Geometry: final body of the model. Coordinates: model frame, mm. Face numbers are marked on the shaded views. A direction names the side the tool comes from. Round coordinates to 2 decimals unless told otherwise and drop trailing zeros. Write each loop counter-clockwise with the first axis right and the second up, starting at its lowest first coordinate (ties: lowest second). Pieces come first, ordered by that corner, then holes. Notation, with made-up numbers: M 63.25,22.5 L 107.25,22.5 A13 cw 107.25,32.5 Z; hole C 55.5,44 d10. An arc over 180 degrees is marked long. Put each result on its own line as item: value. Start each with the question number.
```python
from build123d import *

# Parameters (mm, degrees)
F0_W     = 6
F0_H     = 18
F1_DEPTH = 12
F2_W     = 6
F2_H     = 9
F2_W_2   = 2
F2_H_2   = 4
F3_DEPTH = 10
F4_R     = 1.5
F5_DEPTH = 5


with BuildPart() as f1:
    # F0 (on Top) → F1 (new body)
    with BuildSketch(Plane.XY):
        Rectangle(F0_W, F0_H)
    extrude(amount=F1_DEPTH)

    # F2 (on face) → F3 (cut)
    with BuildSketch(Plane(origin=(0, 0, 0), x_dir=(1, 0, 0), z_dir=(0, 0, -1))):
        with Locations((0, 4.5)):
            Rectangle(F2_W, F2_H)
        with Locations((0, 5.5)):
            Rectangle(F2_W_2, F2_H_2, mode=Mode.SUBTRACT)
    extrude(amount=-F3_DEPTH, mode=Mode.SUBTRACT)

    # F4 (on face) → F5 (join)
    with BuildSketch(Plane(origin=(0, 9, 0), x_dir=(-1, 0, 0), z_dir=(0, 1, 0))):
        with Locations((0, 6)):
            Circle(F4_R)
    extrude(amount=F5_DEPTH)


solid = f1.part
```
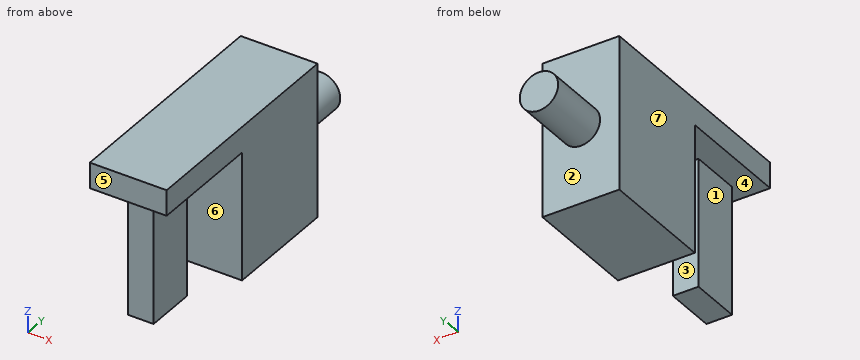
1) Section A-A, the plane z = 6. Output: boundary loops of the cut face in (x, y).
2) First-contact query: pin 1 (1.5 mm diameter, centred on x = 2, z = 6.5, fed in from -Y); pin 2 (1.8 mm diameter, centred on x = -0.5, y = -6.5, fed in from -Z); pin 3 (1.8 mm diameter, centred on x = 0, z = 3, fed in from -Y); pin 4 (1.6 mm diameter, centred on x = 0, z = 3, fed in from +Y). Flat tips, straight axial feed; report the tip coordinate or a pass-through.
3) Draft query along Y for the marked faces 4, 5, 6 and 7. Return one class per face: +Y half, -Y half, draft (parallel to the pull), parting line (faces both ways), or undercut.
4) Ray query, probe 1 along Y at (x, z) = (-0.45, 2.25); probe 2 along Y at (x, z) = (-0.45, 7); probe 3 along Z at (x, y) = (-2.4, -4). Return the intervals inside material, ascending.
5) Access query for the marked faces 1, 2 and 3. Directions: +Z, -Z, +X, -X, +Y, -Y. A direction counts if a zero-diameter tool reaches every point of the face in a straight line with its end or side. Return the directions, or none.
6) Section D-D, the plane z = 4.75. Output: boundary loops of the cut face in (x, y), and give its area (3 significant figures).
7) Section B-B, the plane y = -3.75. Output: boundary loops of the cut face in (x, z).
8) Section C-C, the plane x = 0. Output: boundary loops of the cut face in (y, z).
Solved:
1. outline: M -3,0 L 3,0 L 3,9 L 1.5,9 L 1.5,14 L -1.5,14 L -1.5,9 L -3,9 Z; M -1,-7.5 L 1,-7.5 L 1,-3.5 L -1,-3.5 Z
2. pin 1: stops at y = 0
2. pin 2: stops at z = 0
2. pin 3: stops at y = -7.5
2. pin 4: stops at y = 9
3. face 4: undercut
3. face 5: -Y half
3. face 6: undercut
3. face 7: draft
4. probe 1: y = -7.5 to -3.5, 0 to 9
4. probe 2: y = -7.5 to -3.5, 0 to 14
4. probe 3: z = 10 to 12
5. face 1: -Z, -X, -Y
5. face 2: +Y
5. face 3: -Z, +X, -X
6. outline: M -3,0 L 3,0 L 3,9 L 0.83,9 L 0.83,14 L -0.83,14 L -0.83,9 L -3,9 Z; M -1,-7.5 L 1,-7.5 L 1,-3.5 L -1,-3.5 Z
6. area: 70.3 mm2
7. outline: M -3,10 L -1,10 L -1,0 L 1,0 L 1,10 L 3,10 L 3,12 L -3,12 Z
8. outline: M -9,10 L -7.5,10 L -7.5,0 L -3.5,0 L -3.5,10 L 0,10 L 0,0 L 9,0 L 9,4.5 L 14,4.5 L 14,7.5 L 9,7.5 L 9,12 L -9,12 Z
